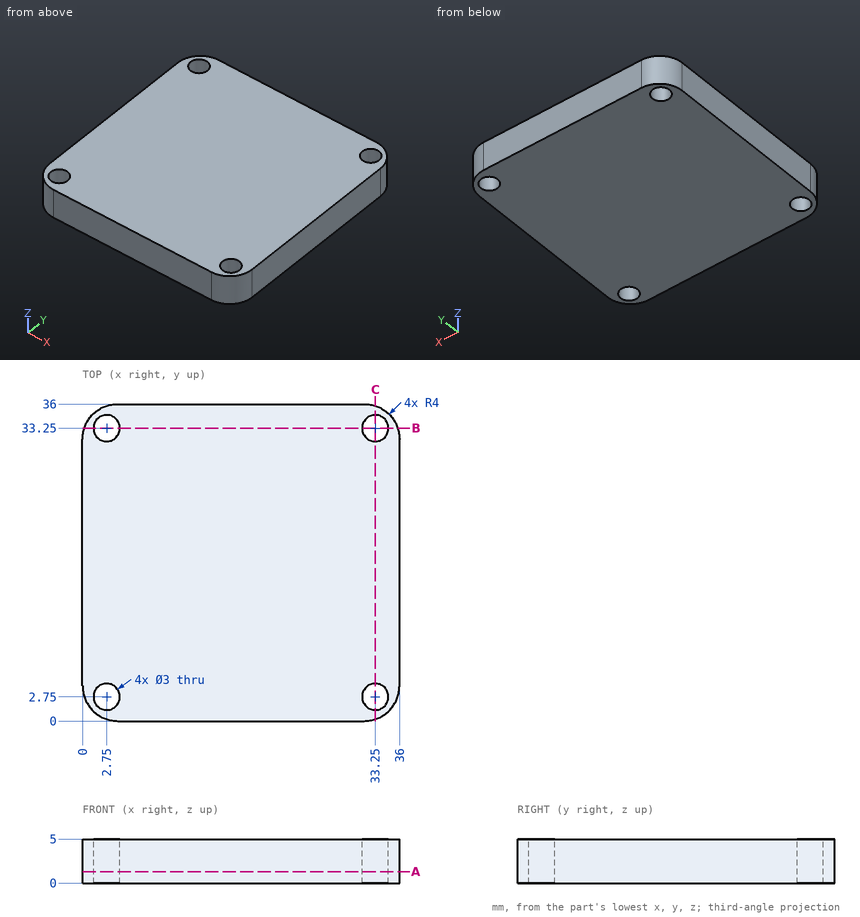
Job drawing, mm, ordinate dimensions from the low corner. One solid piece. Coordinates: 2 decimals unless noted, no trailing zeros. Write each loop counter-clockwise with the first axis right and the second up, starting at its lowest first coordinate (ties: lowest second). Pieces come first, ordered by that corner, then holes. Notation, with made-up numbers: (65, 74.25) -> (108, 74.25) arc R32 cw to (108, 113.25) -> close; hole circle Ø9 at (-35.5, 55.5). An arc over 180 degrees is marked (long way). Use CSV: the item, a comma, the result in double quotes. Start each with the question number.
Item 1: Band-saw the part on A-A, the plane z = 1.3. Write the cut outline in (x, y).
Item 2: Band-saw the part on B-B, the plane y = 33.25. Write the cut outline in (x, z).
Item 3: Wall check: probe 1 along X at (y, z) = (33.25, 1.45); probe 2 along X at (y, z) = (33, 4.15). Give the ranges that are in metal, low to high.
Response values:
1,outline,"(0, 4) arc R4 ccw to (4, 0) -> (32, 0) arc R4 ccw to (36, 4) -> (36, 32) arc R4 ccw to (32, 36) -> (4, 36) arc R4 ccw to (0, 32) -> close; hole circle Ø3 at (2.75, 2.75); hole circle Ø3 at (2.75, 33.25); hole circle Ø3 at (33.25, 2.75); hole circle Ø3 at (33.25, 33.25)"
2,outline,"(0.2, 0) -> (1.25, 0) -> (1.25, 5) -> (0.2, 5) -> close; (4.25, 0) -> (31.75, 0) -> (31.75, 5) -> (4.25, 5) -> close; (34.75, 0) -> (35.8, 0) -> (35.8, 5) -> (34.75, 5) -> close"
3,probe 1,"x = 0.2 to 1.25, 4.25 to 31.75, 34.75 to 35.8"
3,probe 2,"x = 0.13 to 1.27, 4.23 to 31.77, 34.73 to 35.87"
